Geometry check sheet. Reference: the model listing, model coordinates, mm. Coordinates: 2 decimals unless noted, no trailing zeros. Write each loop counter-clockwise with the first axis right and the second up, starting at its lowest first coordinate (ties: lowest second). Pieces come first, ordered by that corner, then holes. Notation, with made-up numbers: (35, 22.5) -> (64, 22.5) arc R21 ccw to (64, 52.5) -> close; hole circle Ø7 at (78, 42.25). An arc over 180 degrees is marked (long way). Use a Markdown table: item, result.
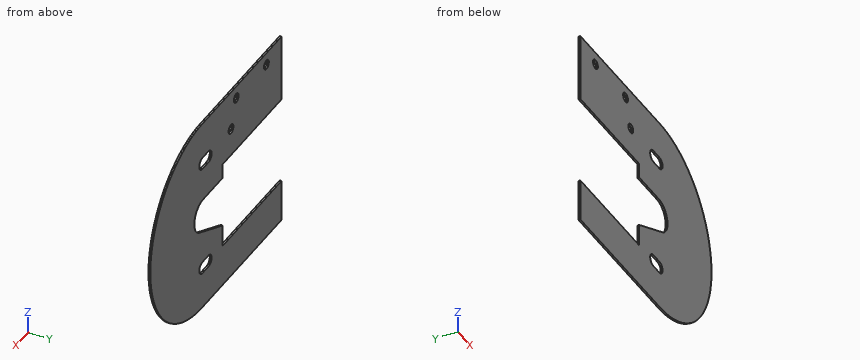
```python
from build123d import *

# Parameters (mm, degrees)
F0_R     = 4.0005
F1_DEPTH = 1.5748


with BuildPart() as f1:
    # F0 (on Front) → F1 (new body)
    with BuildSketch(Plane.XZ):
        with BuildLine():
            Line((732.4313869209, 36.5125), (732.4313869209, 0))
            Line((732.4313869209, 0), (864.6383869209, 0))
            ThreePointArc((864.6383869209, 0), (866.7557920134, 0.0261539128), (868.8719051041, 0.1045996926))
            ThreePointArc((868.8719051041, 0.1045996926), (878.3590689291, 1.1051529768), (887.6763155537, 3.1536401389))
            ThreePointArc((887.6763155537, 3.1536401389), (903.696677756, 9.4149381337), (918.1445842563, 18.748418483))
            ThreePointArc((918.1445842563, 18.748418483), (921.7883869209, 21.8293575429), (925.2551157381, 25.1082711828))
            Line((925.2551157381, 25.1082711828), (873.8802209099, 76.483166011))
            ThreePointArc((873.8802209099, 76.483166011), (871.5444569052, 74.2857554291), (868.7774235028, 72.664665394))
            Line((868.7774235028, 72.664665394), (830.2213869209, 55.5625))
            Line((830.2213869209, 55.5625), (830.2213869209, 36.5125))
            Line((830.2213869209, 36.5125), (747.6713869209, 36.5125))
            Line((747.6713869209, 36.5125), (732.4313869209, 36.5125))
        make_face()
        with BuildLine():
            ThreePointArc((853.6528869209, 31.8135), (848.5093869209, 36.957), (853.6528869209, 42.1005))
            Line((853.6528869209, 42.1005), (863.9398869209, 42.1005))
            ThreePointArc((863.9398869209, 42.1005), (867.57689065, 40.594003729), (869.0833869209, 36.957))
            ThreePointArc((869.0833869209, 36.957), (867.57689065, 33.319996271), (863.9398869209, 31.8135))
            Line((863.9398869209, 31.8135), (853.6528869209, 31.8135))
        make_face(mode=Mode.SUBTRACT)
        with BuildLine():
            Line((732.4313869209, 112.7125), (747.6713869209, 112.7125))
            Line((747.6713869209, 112.7125), (830.2213869209, 112.7125))
            Line((830.2213869209, 112.7125), (830.2213869209, 100.0125))
            Line((830.2213869209, 100.0125), (862.984296866, 100.0125))
            ThreePointArc((862.984296866, 100.0125), (868.9880437433, 98.6898632728), (873.8802209099, 94.966833989))
            Line((873.8802209099, 94.966833989), (925.2551157381, 146.3417288172))
            ThreePointArc((925.2551157381, 146.3417288172), (921.7883869209, 149.6206424571), (918.1445842563, 152.701581517))
            ThreePointArc((918.1445842563, 152.701581517), (901.799905044, 162.9765190517), (883.5704291304, 169.3333333333))
            ThreePointArc((883.5704291304, 169.3333333333), (874.1633869209, 170.9191899427), (864.6383869209, 171.45))
            Line((864.6383869209, 171.45), (858.2883869209, 171.45))
            Line((858.2883869209, 171.45), (839.2383869209, 171.45))
            Line((839.2383869209, 171.45), (749.5336282768, 171.45))
            Line((749.5336282768, 171.45), (732.4313869209, 171.45))
            Line((732.4313869209, 171.45), (732.4313869209, 112.7125))
        make_face()
        with Locations((816.3148869209, 137.033)):
            Circle(F0_R, mode=Mode.SUBTRACT)
        with BuildLine():
            ThreePointArc((853.6528869209, 129.2225), (848.5093869209, 134.366), (853.6528869209, 139.5095))
            Line((853.6528869209, 139.5095), (863.9398869209, 139.5095))
            ThreePointArc((863.9398869209, 139.5095), (867.57689065, 138.003003729), (869.0833869209, 134.366))
            ThreePointArc((869.0833869209, 134.366), (867.57689065, 130.728996271), (863.9398869209, 129.2225))
            Line((863.9398869209, 129.2225), (853.6528869209, 129.2225))
        make_face(mode=Mode.SUBTRACT)
        with Locations((757.5138869209, 160.655)):
            Circle(F0_R, mode=Mode.SUBTRACT)
        with Locations((807.5772869209, 160.655)):
            Circle(F0_R, mode=Mode.SUBTRACT)
        with BuildLine():
            Line((873.8802209099, 76.483166011), (925.2551157381, 25.1082711828))
            ThreePointArc((925.2551157381, 25.1082711828), (928.534029378, 28.575), (931.6149684379, 32.2188026646))
            ThreePointArc((931.6149684379, 32.2188026646), (943.8379598455, 52.9194627605), (949.8325768637, 76.2))
            ThreePointArc((949.8325768637, 76.2), (950.2305815354, 80.9551104752), (950.3633869209, 85.725))
            Line((950.3633869209, 85.725), (877.271796866, 85.725))
            ThreePointArc((877.271796866, 85.725), (876.3971297328, 80.8027473921), (873.8802209099, 76.483166011))
        make_face()
        with BuildLine():
            ThreePointArc((873.8802209099, 94.966833989), (876.3971297328, 90.6472526079), (877.271796866, 85.725))
            Line((877.271796866, 85.725), (950.3633869209, 85.725))
            ThreePointArc((950.3633869209, 85.725), (950.2305815354, 90.4948895248), (949.8325768637, 95.25))
            ThreePointArc((949.8325768637, 95.25), (943.8379598455, 118.5305372395), (931.6149684379, 139.2311973354))
            ThreePointArc((931.6149684379, 139.2311973354), (928.534029378, 142.875), (925.2551157381, 146.3417288172))
            Line((925.2551157381, 146.3417288172), (873.8802209099, 94.966833989))
        make_face()
    extrude(amount=F1_DEPTH)


solid = f1.part
```
Item 1: Section check C-C on z = 122.5. Record the boundary of the cut face in (x, y).
Answer block:
| item | result |
|---|---|
| outline | (732.43, -1.57) -> (942.07, -1.57) -> (942.07, 0) -> (732.43, 0) -> close |
Item 2: Thickness scan on L1, parallel to Z at x = 797, y = -0.7; L2, parallel to X at y = -0.25, z = 135; L3, parallel to Z at x = 760.5, y = -0.85. Record the ranges inside material, lowest first. Write a range as [from, to].
Answer block:
| item | result |
|---|---|
| L1 | z = [0, 36.51], [112.71, 171.45] |
| L2 | x = [732.43, 812.87], [819.76, 848.55], [869.04, 934.79] |
| L3 | z = [0, 36.51], [112.71, 157.99], [163.32, 171.45] |
Item 3: Section check A-A on x = 800. Record the boundary of the cut face in (y, z), then the cut area to 3 significant figures.
Answer block:
| item | result |
|---|---|
| outline | (-1.57, 0) -> (0, 0) -> (0, 36.51) -> (-1.57, 36.51) -> close; (-1.57, 112.71) -> (0, 112.71) -> (0, 171.45) -> (-1.57, 171.45) -> close |
| area | 150 mm^2 |
Item 4: Section check D-D on x = 914.5. Record the boundary of the cut face in (y, z).
Answer block:
| item | result |
|---|---|
| outline | (-1.57, 15.99) -> (0, 15.99) -> (0, 155.46) -> (-1.57, 155.46) -> close |
Item 5: Section check B-B on y = -0.85. Count the separate pieces of the cut face and the enclosed holes in it, then the cut area to 3 significant figures.
Answer block:
| item | result |
|---|---|
| separate pieces | 1 |
| enclosed holes | 5 |
| area | 24,700 mm^2 |
Item 6: Depth check by flat-ended pin: P1, Ø0.8, axis at y = -1, z = 44, coming from the -X side; P2, Ø5, axis at x = 757.51, z = 160.66, coming from the +Y side. Enter the tip coordinate at first touch or a pass-through.
Answer block:
| item | result |
|---|---|
| P1 | stops at x = 830.22 |
| P2 | passes through |
